Can you work these out from the drawing? Everything is in mm from the part's minimum corner. Give positions to 0.01 mm unless a question says otherwise; leave off trailing zeros. Loops run counter-clockwise (first coordinate to the right, second up) from the corner with the lowest first, then second, coordinate; pieces in that order, holes last. Notation, with made-up numbers: M 75,46.5 L 125,46.5 A23 cw 125,59.5 Z; hole C 80.5,45 d5. An arc over 180 degrees is marked long. Use CSV: the item, a comma, the result in double quotes.
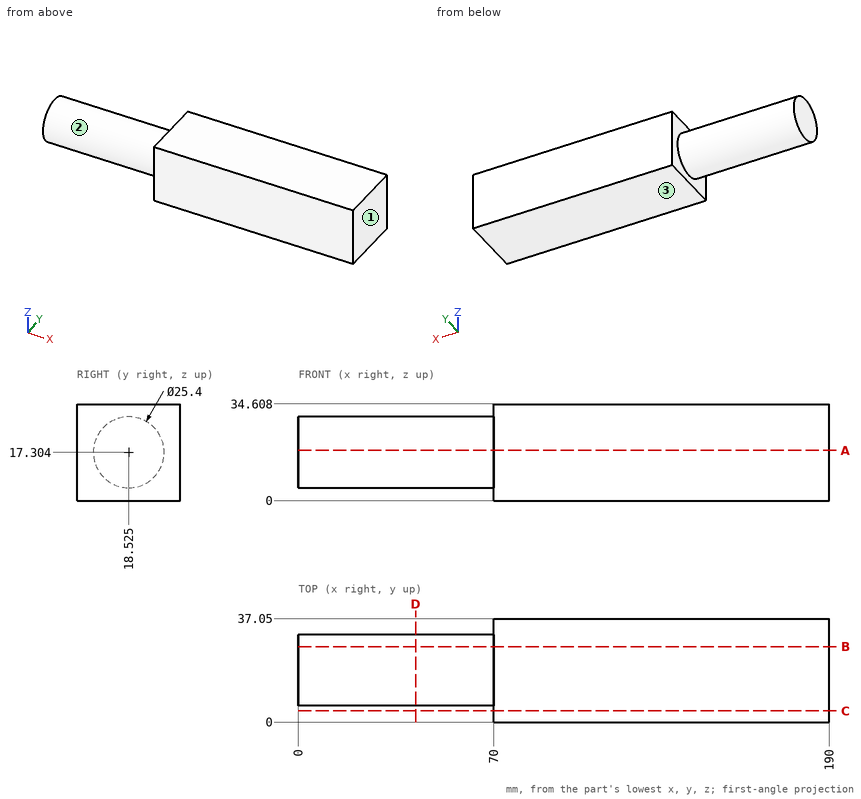
Q1. Please list where these lines run through material, in increasing order: L1, parallel to X at y = 13, z = 2; L2, parallel to Y at x = 66.5, z = 20 (1 decimal); L3, parallel to Y at x = 67.5, z = 28. Write a range as from..to.
Model answer:
L1,"70..190"
L2,"6.1..30.9"
L3,"11.68..25.37"
Q2. I want a section at D-D, the plane x = 42. Please give me the cut outline in (y, z) (1 decimal), then the cut area to 3 significant figures.
Model answer:
outline,"C 18.5,17.3 d25.4"
area,"507 mm2"
Q3. If we mould it in two halves opening along Z, with no side actions, what happens to the marked faces 1, 2 and 3? For each: released by +Z, released by -Z, zero draft, split by the parting line, or undercut.
Model answer:
face 1,"zero draft"
face 2,"split by the parting line"
face 3,"released by -Z"
Q4. I'm going to push a flat-ended pin straight in: P1, Ø2, axis at x = 67, y = 11, coming from the -Z side. Where does the tip first touch, or does it pass through?
Model answer:
P1,"z = 6.41"
Q5. I want a section at C-C, the plane y = 4. Please give me the cut outline in (x, z), then the cut area to 3 significant figures.
Model answer:
outline,"M 70,0 L 190,0 L 190,34.61 L 70,34.61 Z"
area,"4,150 mm2"
Q6. I want a section at B-B, the plane y = 27. Please give me the cut outline in (x, z) (1 decimal).
Model answer:
outline,"M 0,7.8 L 70,7.8 L 70,0 L 190,0 L 190,34.6 L 70,34.6 L 70,26.8 L 0,26.8 Z"
Q7. I want a section at A-A, the plane z = 18. Please give me the cut outline in (x, y).
Model answer:
outline,"M 0,5.84 L 70,5.84 L 70,0 L 190,0 L 190,37.05 L 70,37.05 L 70,31.21 L 0,31.21 Z"
